```python
from build123d import *

# Parameters (mm, degrees)
F0_R      = 40
F1_DEPTH  = 30
F2_W      = 70
F2_H      = 70
F3_DEPTH  = 30
F4_R      = 16
F5_DEPTH  = 60.001
F6_R      = 25
F7_DEPTH  = 7
F8_R      = 2.5
F9_DEPTH  = 25
F10_R     = 3
F11_DEPTH = 25


with BuildPart() as f1:
    # F0 (on Front) → F1 (new body)
    with BuildSketch(Plane.XZ):
        Circle(F0_R)
    extrude(amount=F1_DEPTH)

    # F2 (on face) → F3 (join)
    with BuildSketch(Plane.XZ.offset(30)):
        Rectangle(F2_W, F2_H)
    extrude(amount=F3_DEPTH)

    # F4 (on face) → F5 (cut, through all)
    with BuildSketch(Plane(origin=(0, 0, 0), x_dir=(-1, 0, 0), z_dir=(0, 1, 0))):
        Circle(F4_R)
    extrude(amount=-F5_DEPTH, mode=Mode.SUBTRACT)

    # F6 (on face) → F7 (cut)
    with BuildSketch(Plane(origin=(0, 0, 0), x_dir=(-1, 0, 0), z_dir=(0, 1, 0))):
        Circle(F6_R)
    extrude(amount=-F7_DEPTH, mode=Mode.SUBTRACT)

    # F8 (on face) → F9 (cut)
    with BuildSketch(Plane(origin=(0, 0, 0), x_dir=(-1, 0, 0), z_dir=(0, 1, 0))):
        with Locations((-22.98097, 22.98097)):
            Circle(F8_R)
        with Locations((22.98097, 22.98097)):
            Circle(F8_R)
        with Locations((22.98097, -22.98097)):
            Circle(F8_R)
        with Locations((-22.98097, -22.98097)):
            Circle(F8_R)
    extrude(amount=-F9_DEPTH, mode=Mode.SUBTRACT)

    # F10 (on face) → F11 (cut)
    with BuildSketch(Plane.XZ.offset(60)):
        with Locations((-19.445436, 19.445436)):
            Circle(F10_R)
        with Locations((19.445436, 19.445436)):
            Circle(F10_R)
        with Locations((19.445436, -19.445436)):
            Circle(F10_R)
        with Locations((-19.445436, -19.445436)):
            Circle(F10_R)
    extrude(amount=-F11_DEPTH, mode=Mode.SUBTRACT)


solid = f1.part
```
Design review of the part built by this model. Coordinates are the model's own, in mm. A direction names the side the tool comes from. Coordinates: 2 decimals unless noted, no trailing zeros. Loops run counter-clockwise (first coordinate to the right, second up) from the corner with the lowest first, then second, coordinate; pieces in that order, holes last.
Q1. We need section B-B on z = 0. State the section outline as (x, y) points, and give its area (3 significant figures).
Reported:
outline: (-40, -30) - (-35, -30) - (-35, -60) - (-16, -60) - (-16, -7) - (-25, -7) - (-25, 0) - (-40, 0) - close; (16, -60) - (35, -60) - (35, -30) - (40, -30) - (40, 0) - (25, 0) - (25, -7) - (16, -7) - close
area: 2,450 mm2
Q2. We need section D-D on y = -54. State the section outline as (x, z) points.
Reported:
outline: (-35, -35) - (35, -35) - (35, 35) - (-35, 35) - close; hole circle Ø6 at (-19.45, -19.45); hole circle Ø6 at (-19.45, 19.45); hole circle Ø32 at (0, 0); hole circle Ø6 at (19.45, -19.45); hole circle Ø6 at (19.45, 19.45)
Q3. We need section A-A on x = 0. State the section outline as (y, z) points.
Reported:
outline: (-60, -35) - (-30, -35) - (-30, -40) - (0, -40) - (0, -25) - (-7, -25) - (-7, -16) - (-60, -16) - close; (-60, 16) - (-7, 16) - (-7, 25) - (0, 25) - (0, 40) - (-30, 40) - (-30, 35) - (-60, 35) - close
Q4. For pin 1 (4 mm diameter, centred on x = 38, z = 8.5, fed in from -Y); pin 2 (3 mm diameter, centred on y = -29.5, z = -23.5, fed in from +X); pin 3 (5 mm diameter, centred on y = -17.5, z = 17.5, fed in from -X), all flat-tipped, find the tip position at first contact; note any pin that passes through.
Reported:
pin 1: stops at y = -30
pin 2: stops at x = 35
pin 3: stops at x = -37.08
Q5. To check wall thickness, follow line 1 (X direction, y = -52, z = -21); line 2 (X direction, y = -18, z = -22); line 3 (X direction, y = -21.5, z = -6). State the ranges of each line that lie inside material, in increasing order.
Reported:
line 1: x = -35 to -22.01, -16.88 to 16.88, 22.01 to 35
line 2: x = -33.41 to -25.28, -20.68 to 20.68, 25.28 to 33.41
line 3: x = -39.55 to -14.83, 14.83 to 39.55
Q6. Tool access review of faces 4 (the face through (0, -30, 37)), 5 (the face through (-31, -30, 31)), 6 (the face through (-25.29, -12.32, 22.02)): name each direction out of +Z, -Z, +X, -X, +Y, -Y from which nothing blocks a thin tool from reaching the whole face with its end or side.
Reported:
face 4: +Z, +X, -X, -Y
face 5: +Z, -X, +Y
face 6: +Y
Q7. We need section C-C on y = -31.5. State the section outline as (x, z) points, and give its area (3 significant figures).
Reported:
outline: (-35, -35) - (35, -35) - (35, 35) - (-35, 35) - close; hole circle Ø32 at (0, 0)
area: 4,100 mm2
Q8. The part is to be moulded in two halves that separate along Z. For faces 1 (the face through (-8.67, -14.79, -39.05)), 2 (the face through (0, -45, 35)), 3 (the face through (24.82, -12.32, -21.29)), say which applies: +Z half, -Z half, draft (parallel to the pull), parting line (faces both ways), or undercut.
Reported:
face 1: parting line
face 2: +Z half
face 3: undercut
